Read the model definition and answer for the solid it produces. Units are mm, in the model's axes. A direction names the side the tool comes from. Give positions to 0.01 mm unless a question says otherwise; leave off trailing zeros. Order: outer loops, then holes, each group sorted by start corner. A loop starts at its lowest first (then second) coordinate and runs counter-clockwise, first axis right, second up. Notation, with made-up numbers: (76, 54) -> (100, 54) arc R26 ccw to (100, 71) -> close; hole circle Ø2 at (5.5, 63). An arc over 180 degrees is marked (long way). One line per question, with ' | ' between items. Start each with the question number.
```python
from build123d import *

# Parameters (mm, degrees)
SZKIC1_W                    = 100
SZKIC1_H                    = 100
DODANIE_WYCI_GNI_CIE1_DEPTH = 4
SZKIC2_W                    = 3
SZKIC2_H                    = 100
DODANIE_WYCI_GNI_CIE2_DEPTH = 196


with BuildPart() as part:
    # Szkic1 → Dodanie-wyciągnięcie1 (new body)
    with BuildSketch(Plane.XY):
        with Locations((-50, 50)):
            Rectangle(SZKIC1_W, SZKIC1_H)
        with Locations((50, 50)):
            Rectangle(SZKIC1_W, SZKIC1_H)
        with Locations((50, -50)):
            Rectangle(SZKIC1_W, SZKIC1_H)
        with Locations((-50, -50)):
            Rectangle(SZKIC1_W, SZKIC1_H)
    extrude(amount=DODANIE_WYCI_GNI_CIE1_DEPTH)

    # Szkic2 → Dodanie-wyciągnięcie2 (add)
    with BuildSketch(Plane.XY.offset(4)):
        with Locations((-1.5, 50)):
            Rectangle(SZKIC2_W, SZKIC2_H)
        with Locations((1.5, 50)):
            Rectangle(SZKIC2_W, SZKIC2_H)
        with Locations((-1.5, -50)):
            Rectangle(SZKIC2_W, SZKIC2_H)
        with Locations((1.5, -50)):
            Rectangle(SZKIC2_W, SZKIC2_H)
    extrude(amount=DODANIE_WYCI_GNI_CIE2_DEPTH)


solid = part.part
```
Q1. A cutting plane is placed at B-B, the plane x = 52.5. Determine the outline of the cut face in (y, z).
Q2. A cutting plane is placed at A-A, the plane y = 74. Determine the outline of the cut face in (x, z).
Q3. Given P1, Ø5, axis at y = -43, z = 24.5, coming from the -X side; P2, Ø8, axis at x = 40, y = -55, coming from the +Z side, each flat-ended and moving along its own axis, determine where each tip first touches the part or whether it passes through.
Q4. A cutting plane is placed at C-C, the plane z = 175.5. Determine the outline of the cut face in (x, y), then the cut area to 3 significant figures.
Q5. Find the intervals of material crossed by line 1 (Z direction, x = 55.5, y = -75.5); line 2 (X direction, y = 17, z = 168), in increasing order.
Q6. Which of the six approach directions +Z, -Z, +X, -X, +Y, -Y give full straight-line access (tool end or side, diameter ignored) to faces 1 (the flat face through (51, 1, 4)), 2 (the flat face through (-52, 1, 4)), 3 (the flat face through (-1, 1, 0))?
Geometry results:
1) outline: (-100, 0) -> (100, 0) -> (100, 4) -> (-100, 4) -> close
2) outline: (-100, 0) -> (100, 0) -> (100, 4) -> (3, 4) -> (3, 200) -> (-3, 200) -> (-3, 4) -> (-100, 4) -> close
3) P1: x = -3 | P2: z = 4
4) outline: (-3, -100) -> (3, -100) -> (3, 100) -> (-3, 100) -> close | area: 1,200 mm²
5) line 1: 0 to 4 | line 2: -3 to 3
6) face 1: +Z, +X, +Y, -Y | face 2: +Z, -X, +Y, -Y | face 3: -Z, +X, -X, +Y, -Y
